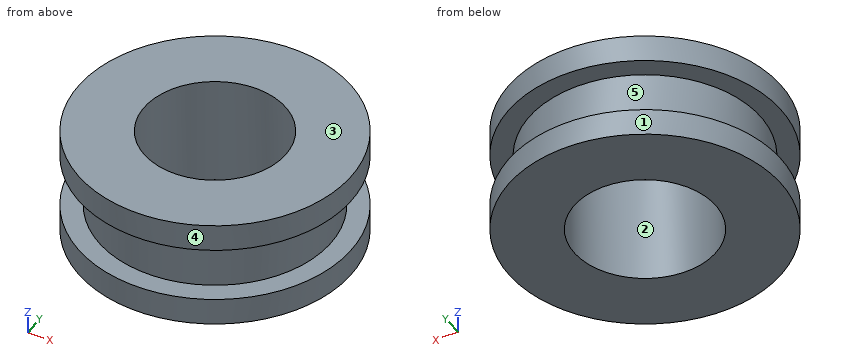
```python
from build123d import *

# Parameters (mm, degrees)
F0_R     = 5
F1_DEPTH = 4
F3_R     = 5
F3_R_2   = 4.25
F4_DEPTH = 3
F2_R     = 2.6
F5_DEPTH = 4.001
F6_DEPTH = 1


with BuildPart() as f1:
    # F0 (on Top) → F1 (new body)
    with BuildSketch(Plane.XY):
        Circle(F0_R)
    extrude(amount=F1_DEPTH)

    # F3 (on face) → F4 (cut)
    with BuildSketch(Plane(origin=(0, 0, 0), x_dir=(1, 0, 0), z_dir=(0, 0, -1))):
        Circle(F3_R)
        Circle(F3_R_2, mode=Mode.SUBTRACT)
    extrude(amount=-F4_DEPTH, mode=Mode.SUBTRACT)

    # F2 (on face) → F5 (cut, through all)
    with BuildSketch(Plane.XY.offset(4)):
        Circle(F2_R)
    extrude(amount=-F5_DEPTH, mode=Mode.SUBTRACT)

    # F3 (on face) → F6 (join)
    with BuildSketch(Plane(origin=(0, 0, 0), x_dir=(1, 0, 0), z_dir=(0, 0, -1))):
        Circle(F3_R)
        Circle(F3_R_2, mode=Mode.SUBTRACT)
    extrude(amount=-F6_DEPTH)


solid = f1.part
```
Model file for the job. Use its own axes, mm. Face numbers are marked on the shaded views. A direction names the side the tool comes from. Coordinates: 2 decimals unless noted, no trailing zeros. Loops run counter-clockwise (first coordinate to the right, second up) from the corner with the lowest first, then second, coordinate; pieces in that order, holes last. Notation, with made-up numbers: M 80,81.5 L 111,81.5 A28 cw 111,108.5 Z; hole C 21.25,76 d9. An arc over 180 degrees is marked long. Use CSV: the item, a comma, the result in double quotes. Start each with the question number.
1. Flat gauge pin, fed straight in: pin 1 (3 mm diameter, centred on x = 0, y = 0, fed in from +Z). Where does the tip first touch, or does it go through?
2. Band-saw the part on D-D, the plane x = -2.75. List the corners of the cut face in (y, z), then the cut area to 3 significant figures.
3. Two-plate mould, pull along X, no slides. Class the marked faces 1, 2 and 3: pulls with the +X half, pulls with the -X half, needs draft (parallel to the pull), parting line crosses it, or undercut.
4. Probe probe 1 along Z at (x, y) = (-3, 3.75); probe 2 along Y at (x, z) = (0, 1.3); probe 3 along Y at (x, z) = (-2.25, 1.8). List the from-to ranges inside material, lowest first. Write a range as [from, to].
5. Band-saw the part on A-A, the plane x = 0. List the corners of the cut face in (y, z).
6. Band-saw the part on C-C, the plane z = 2. List the corners of the cut face in (x, y).
7. Tool access for the marked faces 4 and 5: list every direction of +Z, -Z, +X, -X, +Y, -Y with a clear straight run to the whole face (end or side of a thin tool).
Entries:
1,pin 1,"passes through"
2,outline,"M -4.18,0 L 4.18,0 L 4.18,1 L 3.24,1 L 3.24,3 L 4.18,3 L 4.18,4 L -4.18,4 L -4.18,3 L -3.24,3 L -3.24,1 L -4.18,1 Z"
2,area,"29.7 mm2"
3,face 1,"parting line crosses it"
3,face 2,"undercut"
3,face 3,"needs draft"
4,probe 1,"z = [0, 1], [3, 4]"
4,probe 2,"y = [-4.25, -2.6], [2.6, 4.25]"
4,probe 3,"y = [-3.61, -1.3], [1.3, 3.61]"
5,outline,"M -5,0 L -2.6,0 L -2.6,4 L -5,4 L -5,3 L -4.25,3 L -4.25,1 L -5,1 Z; M 2.6,0 L 5,0 L 5,1 L 4.25,1 L 4.25,3 L 5,3 L 5,4 L 2.6,4 Z"
6,outline,"C 0,0 d8.5; hole C 0,0 d5.2"
7,face 4,"+Z, -Z"
7,face 5,"none"
